```python
from build123d import *

# Parameters (mm, degrees)
F0_W     = 125.33
F0_H     = 74.41
F1_DEPTH = 2
F2_W     = 121.01
F2_H     = 70.09
F2_W_2   = 117.01
F2_H_2   = 66.09
F3_DEPTH = 6
F4_R     = 1.5
F5_DEPTH = 8.001


with BuildPart() as f1:
    # F0 (on Top) → F1 (new body)
    with BuildSketch(Plane.XY):
        Rectangle(F0_W, F0_H)
    extrude(amount=F1_DEPTH)

    # F2 (on face) → F3 (join)
    with BuildSketch(Plane.XY.offset(2)):
        Rectangle(F2_W, F2_H)
        Rectangle(F2_W_2, F2_H_2, mode=Mode.SUBTRACT)
    extrude(amount=F3_DEPTH)

    # F4 (on face) → F5 (cut, through all)
    with BuildSketch(Plane(origin=(0, 0, 0), x_dir=(1, 0, 0), z_dir=(0, 0, -1))):
        with Locations((-39.435246, 14.143545)):
            Circle(F4_R)
        with Locations((-35.077156, 16.39686)):
            Circle(F4_R)
        with Locations((-31.077552, 18.983332)):
            Circle(F4_R)
        with Locations((-29.828973, 13.146486)):
            Circle(F4_R)
        with Locations((-32.249665, 7.690482)):
            Circle(F4_R)
        with Locations((-35.304773, 11.495986)):
            Circle(F4_R)
        with Locations((-37.415004, 4.699329)):
            Circle(F4_R)
        with Locations((-43.352007, 5.315545)):
            Circle(F4_R)
        with Locations((-39.662862, 9.242671)):
            Circle(F4_R)
        with Locations((-39.20763, 19.044419)):
            Circle(F4_R)
        with Locations((-35.518485, 22.971545)):
            Circle(F4_R)
        with Locations((-41.455488, 23.587761)):
            Circle(F4_R)
        with Locations((-46.620827, 20.596608)):
            Circle(F4_R)
        with Locations((-43.565719, 16.791103)):
            Circle(F4_R)
        with Locations((-43.793336, 11.890229)):
            Circle(F4_R)
        with Locations((-47.79294, 9.303757)):
            Circle(F4_R)
        with Locations((-49.041518, 15.140604)):
            Circle(F4_R)
    extrude(amount=-F5_DEPTH, mode=Mode.SUBTRACT)


solid = f1.part
```
Geometry: final body of the model. Coordinates: model frame, mm. A direction names the side the tool comes from. Coordinates: 2 decimals unless noted, no trailing zeros. Order: outer loops, then holes, each group sorted by start corner. A loop starts at its lowest first (then second) coordinate and runs counter-clockwise, first axis right, second up. Notation, with made-up numbers: (0.5, -31) -> (47.5, -31) arc R21 ccw to (47.5, -14) -> close; hole circle Ø1 at (-9.75, -14). An arc over 180 degrees is marked (long way). Use CSV: the item, a comma, the result in double quotes.
1) Access query for faces 3 (the flat face through (-58.505, 0, 5)), 4 (the cylindrical face through (-42.56, -24.6, 0.99)), 5 (the flat face through (-1, 35.045, 5)). Directions: +Z, -Z, +X, -X, +Y, -Y. A direction counts if a zero-diameter tool reaches every point of the face in a straight line with its end or side. Return the directions, or none.
Findings:
face 3,"+Z"
face 4,"+Z, -Z"
face 5,"+Z, +X, -X, +Y"
2) Section C-C on y = 13. Output: boundary loops of the cut face in (x, z) (3 decimals), then the cut area to 3 significant figures.
Findings:
outline,"(-62.665, 0) -> (62.665, 0) -> (62.665, 2) -> (60.505, 2) -> (60.505, 8) -> (58.505, 8) -> (58.505, 2) -> (-58.505, 2) -> (-58.505, 8) -> (-60.505, 8) -> (-60.505, 2) -> (-62.665, 2) -> close"
area,"275 mm^2"
3) Section A-A on x = -25.5. Output: boundary loops of the cut face in (y, z) (3 decimals), then the cut area to 3 significant figures.
Findings:
outline,"(-37.205, 0) -> (37.205, 0) -> (37.205, 2) -> (35.045, 2) -> (35.045, 8) -> (33.045, 8) -> (33.045, 2) -> (-33.045, 2) -> (-33.045, 8) -> (-35.045, 8) -> (-35.045, 2) -> (-37.205, 2) -> close"
area,"173 mm^2"
4) Line query: line 1 (X direction, y = 20.5, z = 3) (3 decimals); line 2 (Y direction, x = 45, z = 5) (3 decimals); line 3 (Z direction, x = 1, y = 21). Output: solid intervals per line, ascending.
Findings:
line 1,"x = -60.505 to -58.505, 58.505 to 60.505"
line 2,"y = -35.045 to -33.045, 33.045 to 35.045"
line 3,"z = 0 to 2"
5) Mould query, pull axis X, two halves, no side actions, for faces 1 (the flat face through (-1, -33.045, 5)), 2 (the flat face through (-1, 1, 0)). Classes: +X half, -X half, draft (parallel to the pull), parting line (faces both ways), or undercut.
Findings:
face 1,"undercut"
face 2,"draft"
6) Section B-B on z = 3.5. Output: boundary loops of the cut face in (x, y) (3 decimals), then the cut area to 3 significant figures.
Findings:
outline,"(-60.505, -35.045) -> (60.505, -35.045) -> (60.505, 35.045) -> (-60.505, 35.045) -> close; hole (-58.505, -33.045) -> (58.505, -33.045) -> (58.505, 33.045) -> (-58.505, 33.045) -> close"
area,"748 mm^2"
7) Pin query (flat end, axial travel): pin 1 Ø10 at (x, y) = (-37, 5) entering from +Z; pin 2 Ø1.8 at (y, z) = (-6, 4.5) entering from -X (3 decimals); pin 3 Ø2.5 at (x, y) = (-35.3, -11.5) entering from +Z; pin 4 Ø1 at (y, z) = (19.5, 3.5) entering from +X (3 decimals). Return the tip coordinate at first contact, or that it passes through.
Findings:
pin 1,"stops at z = 2"
pin 2,"stops at x = -60.505"
pin 3,"passes through"
pin 4,"stops at x = 60.505"
